Could you check a few things on this model? Use its own coordinates, in mm. A direction names the side the tool comes from. Coordinates: 2 decimals unless noted, no trailing zeros. Order: outer loops, then holes, each group sorted by start corner. A loop starts at its lowest first (then second) coordinate and runs counter-clockwise, first axis right, second up. Notation, with made-up numbers: (73.5, 87) -> (110.5, 87) arc R22 cw to (110.5, 97) -> close; hole circle Ø8 at (55.25, 74.5). An arc over 180 degrees is marked (long way). Use a Markdown table: item, result. Add a question column.
1) If we section it at A-A (x = 15.75): Write out the boundary of the cut face in (y, z) (3 decimals), plus the area to 3 significant figures.
2) If we section it at C-C (z = 101.6): Write out the boundary of the cut face in (x, y) (3 decimals), plus the area to 3 significant figures.
3) Thinking about a two-plate mould opening in X: for faces 3 (the flat face through (24, 13, 355.6)), 4 (the flat face through (22.225, 13, 175)), 5 (the flat face through (25.4, 13, 175)), 6 (the flat face through (13, 22.225, 175)), which applies, +X half, -X half, draft (parallel to the pull), parting line (faces both ways), or undercut?
4) If we section it at D-D (z = 277): Write out the boundary of the cut face in (x, y) (3 decimals).
5) Will this pin go through, and if not, where does the flat tip stop? pin 1 Ø3 at (x, y) = (20.5, 16) entering from -Z.
6) If I drill on L1, parallel to X at y = 22, z = 20 (3 decimals); L2, parallel to Z at x = 1.35, y = 12.7 (3 decimals), over which ranges is the centre line in solid material (lowest first)? Write a range as [from, to].
7) Which directions (+Z, -Z, +X, -X, +Y, -Y) give clear straight access to the entire face, cutting with the end or side of a thin tool? Please do faces 1 (the flat face through (13, 25.4, 175)), 2 (the flat face through (13, 3.175, 175)).
8) If we section it at B-B (y = 12.7): Write out the boundary of the cut face in (x, z) (3 decimals).
```python
from build123d import *

# Parameters (mm, degrees)
SKETCH1_W           = 25.4
SKETCH1_H           = 25.4
SKETCH1_W_2         = 19.05
SKETCH1_H_2         = 19.05
BOSS_EXTRUDE1_DEPTH = 355.6
SKETCH2_R           = 3.175
CUT_EXTRUDE1_DEPTH  = 358.409680899


with BuildPart() as part:
    # Sketch1 → Boss-Extrude1 (new body)
    with BuildSketch(Plane.XY):
        with Locations((12.7, 12.7)):
            Rectangle(SKETCH1_W, SKETCH1_H)
        with Locations((12.7, 12.7)):
            Rectangle(SKETCH1_W_2, SKETCH1_H_2, mode=Mode.SUBTRACT)
    extrude(amount=BOSS_EXTRUDE1_DEPTH)

    # Sketch2 → Cut-Extrude1 (cut, through all)
    with BuildSketch(Plane.ZY):
        with Locations(Location((101.6, 12.7, 0), (0, 0, 270))):
            Circle(SKETCH2_R)
    extrude(amount=-CUT_EXTRUDE1_DEPTH, mode=Mode.SUBTRACT)


solid = part.part
```
Answer sheet:
| question | item | result |
|---|---|---|
| 1 | outline | (0, 0) -> (3.175, 0) -> (3.175, 355.6) -> (0, 355.6) -> close; (22.225, 0) -> (25.4, 0) -> (25.4, 355.6) -> (22.225, 355.6) -> close |
| 1 | area | 2,260 mm2 |
| 2 | outline | (0, 0) -> (25.4, 0) -> (25.4, 9.525) -> (22.225, 9.525) -> (22.225, 3.175) -> (3.175, 3.175) -> (3.175, 9.525) -> (0, 9.525) -> close; (0, 15.875) -> (3.175, 15.875) -> (3.175, 22.225) -> (22.225, 22.225) -> (22.225, 15.875) -> (25.4, 15.875) -> (25.4, 25.4) -> (0, 25.4) -> close |
| 2 | area | 242 mm2 |
| 3 | face 3 | draft |
| 3 | face 4 | undercut |
| 3 | face 5 | +X half |
| 3 | face 6 | undercut |
| 4 | outline | (0, 0) -> (25.4, 0) -> (25.4, 25.4) -> (0, 25.4) -> close; hole (3.175, 3.175) -> (22.225, 3.175) -> (22.225, 22.225) -> (3.175, 22.225) -> close |
| 5 | pin 1 | through |
| 6 | L1 | [0, 3.175], [22.225, 25.4] |
| 6 | L2 | [0, 98.425], [104.775, 355.6] |
| 7 | face 1 | +Z, -Z, +X, -X, +Y |
| 7 | face 2 | +Z, -Z |
| 8 | outline | (0, 0) -> (3.175, 0) -> (3.175, 98.425) -> (0, 98.425) -> close; (0, 104.775) -> (3.175, 104.775) -> (3.175, 355.6) -> (0, 355.6) -> close; (22.225, 0) -> (25.4, 0) -> (25.4, 98.425) -> (22.225, 98.425) -> close; (22.225, 104.775) -> (25.4, 104.775) -> (25.4, 355.6) -> (22.225, 355.6) -> close |
